Check sheet for the modelled part. Datum: model origin and axes. Units: mm. Face numbers are marked on the shaded views. A direction names the side the tool comes from. Give positions to 0.01 mm unless a question says otherwise; leave off trailing zeros. Write each loop counter-clockwise with the first axis right and the second up, starting at its lowest first coordinate (ties: lowest second). Pieces come first, ordered by that corner, then holes. Notation, with made-up numbers: (-4, 10) -> (40, 10) arc R10 cw to (40, 22) -> close; hole circle Ø8 at (-38, 79). An arc over 180 degrees is marked (long way). Use a Markdown table: item, result. Add a question column.
1. Scan lines: probe 1 along X at (y, z) = (127, 9.25); probe 2 along X at (y, z) = (116.5, 8.25); probe 3 along X at (y, z) = (46.5, 7.75). Record each from-to range of solid material in increasing order. Write a range as [from, to].
2. Cross-section at B-B (y = -4.5). Enter the section's corners in (x, z), then the cut area to 3 significant figures.
3. Gauge pin test, flat ends, axial feed: P1, Ø2, axis at x = -71, y = -104, coming from the -Z side; P2, Ø6, axis at y = 212, z = 12.5, coming from the +X side; P3, Ø8, axis at y = -87, z = 16.5, coming from the -X side; P4, Ø2, axis at y = -91, z = 4, coming from the -X side. Record the tip position at first contact, or that the pin passes through.
4. Release check for a two-part mould opening along Y. For the marked faces 3, 4 and 5 record: released by +Y, released by -Y, zero draft, split by the parting line, or undercut.
5. Set-up check for the marked faces 1 and 2: record each of +Z, -Z, +X, -X, +Y, -Y from which the full face is reachable in a straight line by a thin tool's end or side.
6. Cross-section at A-A (x = -45). Enter the section's corners in (y, z).
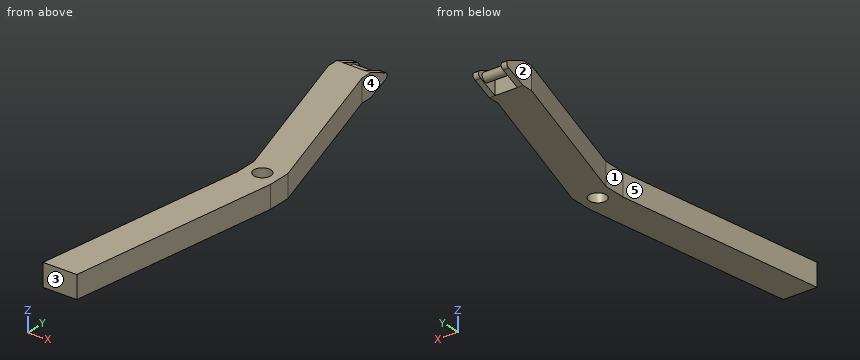
Solid Edge part; units mm, degrees
sketch "Sketch1" plane through (0, 0, 0) normal (0, 0, 1) x (1, 0, 0)
  circle A0 centre (-43.4214, 44.1158) radius 7.5
  line L0 (-103.4214, 199.1158) -> (-58.4214, 54.1158)
  line L1 (-58.4214, 54.1158) -> (-58.4214, 34.1158)
  line L2 (-58.4214, 34.1158) -> (-85.1518, -155.8842)
  line L3 (-85.1518, -155.8842) -> (-55.1518, -155.8842)
  line L4 (-55.1518, -155.8842) -> (-28.4214, 34.1158)
  line L5 (-28.4214, 54.1158) -> (-28.4214, 34.1158)
  line L6 (-73.4214, 199.1158) -> (-28.4214, 54.1158)
  line L7 (-73.4214, 209.1158) -> (-73.4214, 199.1158)
  line L8 (-103.4214, 209.1158) -> (-73.4214, 209.1158)
  line L9 (-103.4214, 199.1158) -> (-103.4214, 209.1158)
  dimension "D1" = 58.4214
  dimension "D2" = 103.4214
  dimension "D3" = 103.4214
  dimension "D4" = 73.4214
  dimension "D5" = 28.4214
  dimension "D6" = 43.4214
extrude "Protrusion1" add sketch "Sketch1" along normal blind 20
sketch "Sketch2" plane through (-73.4214, 6.6158, 20) normal (1, 0, 0) x (0, 0, 1)
  line L0 (-20, -202.5) -> (-13.0975, -218.8561)
  arc A0 (-13.0975, -218.8561) -> (-6.9885, -218.8196) centre (-10.046, -218.3277) ccw
  line L1 (-6.9885, -218.8196) -> (0, -202.5)
  line L2 (-20, -202.5) -> (0, -202.5)
extrude "ExtrudedProtrusion_3" add sketch "Sketch2" against normal blind 5
sketch "Sketch3" plane through (-103.4214, 204.1158, 10) normal (-1, 0, 0) x (0, 1, 0)
  line L0 (5, 10) -> (21.3561, 3.0975)
  arc A0 (21.3561, 3.0975) -> (21.3196, -3.0115) centre (20.7972, 0.0462) cw
  line L1 (5, -10) -> (21.3196, -3.0115)
  line L2 (5, 10) -> (5, -10)
extrude "ExtrudedProtrusion_7" add sketch "Sketch3" against normal blind 5
sketch "Sketch4" plane through (-78.4214, 219.9429, 5) normal (-1, 0, 0) x (0, 0.9213, 0.3888)
  circle A0 centre (1.9464, -4.536) radius 4
extrude "Protrusion2" add sketch "Sketch4" along normal up to vertex (20 mm away)
Worked answers:
| question | item | result |
|---|---|---|
| 1 | probe 1 | x = [-81.04, -51.04] |
| 1 | probe 2 | x = [-77.78, -47.78] |
| 1 | probe 3 | x = [-58.42, -50.53], [-36.31, -28.42] |
| 2 | outline | (-63.85, 0) -> (-33.85, 0) -> (-33.85, 20) -> (-63.85, 20) -> close |
| 2 | area | 600 mm² |
| 3 | P1 | stops at z = 0 |
| 3 | P2 | stops at x = -73.42 |
| 3 | P3 | stops at x = -76.02 |
| 3 | P4 | stops at x = -76.16 |
| 4 | face 3 | released by -Y |
| 4 | face 4 | zero draft |
| 4 | face 5 | undercut |
| 5 | face 1 | +Z, -Z, -X |
| 5 | face 2 | +Z, -Z, -X, +Y, -Y |
| 6 | outline | (-83.73, 0) -> (36.78, 0) -> (36.78, 20) -> (-83.73, 20) -> close; (51.45, 0) -> (107.54, 0) -> (107.54, 20) -> (51.45, 20) -> close |
